Build history of the part. All positions in model axes, mm. Face numbers are marked on the shaded views. A direction names the side the tool comes from. Give positions to 0.01 mm unless a question says otherwise; leave off trailing zeros. Loops run counter-clockwise (first coordinate to the right, second up) from the corner with the lowest first, then second, coordinate; pieces in that order, holes last. Notation, with made-up numbers: M 17.25,33 L 67.25,33 A16 cw 67.25,44 Z; hole C 9,10.5 d7. An arc over 180 degrees is marked long. Answer in a Markdown table with one row per item. Add a question column.
```python
from build123d import *

# Parameters (mm, degrees)
F1_DEPTH = 220
F3_D     = 12.7
F5_D     = 7.62
F7_D     = 12.7


with BuildPart() as f1:
    # F0 (on Front) → F1 (new body)
    with BuildSketch(Plane.XZ):
        Polygon((0, 0), (0, -30), (2, -30), (2, 2), (-48, 2), (-48, 202), (-50, 202), (-50, 0), align=None)
    extrude(amount=F1_DEPTH)

    # F3 (through all)
    with Locations(Plane.YZ.offset(2)):
        with Locations((-169.2, -18.051046), (-50.8, -18.051046)):
            Hole(F3_D / 2)

    # F5 (through all)
    with Locations(Plane.YZ.offset(-48)):
        with Locations((-166.5, 182), (-36.5, 182), (-36.5, 22), (-166.5, 22)):
            Hole(F5_D / 2)

    # F7 (through all)
    with Locations(Plane.XY.offset(2)):
        with Locations((-23, -25.4), (-23, -194.6)):
            Hole(F7_D / 2)


solid = f1.part
```
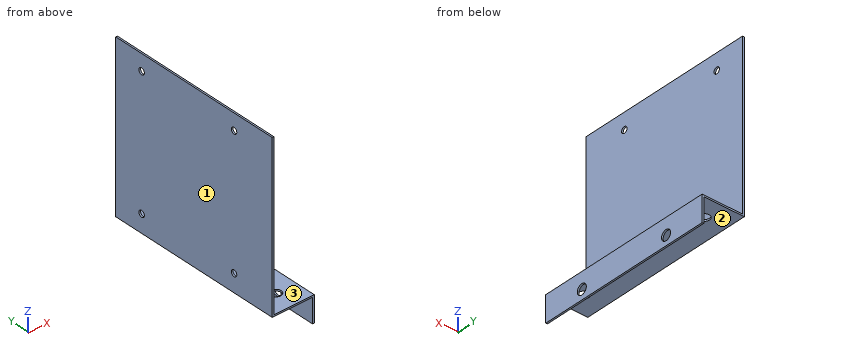
(1) Tool access for the marked faces 1, 2 and 3: list every direction of +Z, -Z, +X, -X, +Y, -Y with a clear straight run to the whole face (end or side of a thin tool).
(2) Wall check: line 1 (Z direction, x = -49.3, y = -166.5); line 2 (Y direction, x = -23, z = 1); line 3 (Y direction, x = -49.25, z = 182). Give the ranges that are in metal, low to high.
(3) Slice it at C-C, the plane z = 22. Give the cut face in (x, y), then the cut area to 3 significant figures.
(4) Slice it at A-A, the plane y = -50.8. Give the cut face in (x, z), then the cut area to 3 significant figures.
(5) Slice it at D-D, the plane y = -166.5. Give the cut face in (x, z), then the cut area to 3 significant figures.
(6) Slice it at B-B, the plane x = -23. Give the cut face in (y, z).
(7) Pin check, flat tips, straight feed: pin 1 (15 mm diameter, centred on x = -25.5, y = -155.5, fed in from -Z); pin 2 (7 mm diameter, centred on y = -36.5, z = 182, fed in from +X); pin 3 (9 mm diameter, centred on y = -99, z = -11, fed in from -X); pin 4 (6 mm diameter, centred on x = -43.5, y = -77.5, fed in from +Z). Stop position of each tip, or through.
Solution:
| question | item | result |
|---|---|---|
| 1 | face 1 | +Z, -Z, -X, +Y, -Y |
| 1 | face 2 | -Z, -X, +Y, -Y |
| 1 | face 3 | +Z, +X, +Y, -Y |
| 2 | line 1 | 0 to 18.19, 25.81 to 178.19, 185.81 to 202 |
| 2 | line 2 | -220 to -200.95, -188.25 to -31.75, -19.05 to 0 |
| 2 | line 3 | -220 to -170.31, -162.69 to -40.31, -32.69 to 0 |
| 3 | outline | M -50,-220 L -48,-220 L -48,-170.31 L -50,-170.31 Z; M -50,-162.69 L -48,-162.69 L -48,-40.31 L -50,-40.31 Z; M -50,-32.69 L -48,-32.69 L -48,0 L -50,0 Z |
| 3 | area | 410 mm^2 |
| 4 | outline | M -50,0 L 0,0 L 0,-11.7 L 2,-11.7 L 2,2 L -48,2 L -48,202 L -50,202 Z; M 0,-30 L 2,-30 L 2,-24.4 L 0,-24.4 Z |
| 4 | area | 539 mm^2 |
| 5 | outline | M -50,0 L 0,0 L 0,-12.3 L 2,-12.3 L 2,2 L -48,2 L -48,18.19 L -50,18.19 Z; M -50,25.81 L -48,25.81 L -48,178.19 L -50,178.19 Z; M -50,185.81 L -48,185.81 L -48,202 L -50,202 Z; M 0,-30 L 2,-30 L 2,-23.8 L 0,-23.8 Z |
| 5 | area | 511 mm^2 |
| 6 | outline | M -220,0 L -200.95,0 L -200.95,2 L -220,2 Z; M -188.25,0 L -31.75,0 L -31.75,2 L -188.25,2 Z; M -19.05,0 L 0,0 L 0,2 L -19.05,2 Z |
| 7 | pin 1 | z = 0 |
| 7 | pin 2 | through |
| 7 | pin 3 | x = 0 |
| 7 | pin 4 | z = 2 |
